Here's how the part is built. I have some questions about the finished solid (model axes, mm). A direction names the side the tool comes from. Round coordinates to 2 decimals unless told otherwise and drop trailing zeros. Order: outer loops, then holes, each group sorted by start corner. A loop starts at its lowest first (then second) coordinate and runs counter-clockwise, first axis right, second up. Notation, with made-up numbers: M 29.5,-16 L 67.5,-16 A17 ccw 67.5,10 Z; hole C -39.75,21 d6. An arc over 180 degrees is marked long. Write item = value, one per line. Start each with the question number.
Item 1: I'm going to push flat-ended pins straight in: P1, Ø6, axis at x = 5, y = 16.5, coming from the -Z side; P2, Ø5.5, axis at x = 0.5, y = 2, coming from the +Z side; P3, Ø5.5, axis at x = -1, z = -1.5, coming from the -Y side. Where does each tip first touch, or does it pass through?
Item 2: Please list where these lines run through material, in increasing order: L1, parallel to X at y = 16.25, z = 0 (3 decimals); L2, parallel to Z at x = -20.5, y = 2; L3, parallel to Y at x = 4, z = -19.
Item 3: For faces 1 (the face through (-2.76, 16.94, -8.75)), 2 (the face through (0, 2, 5.556)), 3 (the face through (-20, 5, 15)), which set-ups out of +Z, -Z, +X, -X, +Y, -Y let a thin tool reach every point of the face, with its end or its side?
Item 4: I want a section at B-B, the plane y = 1.75. List the corners of the cut face in (x, z) for me, plus the area to 3 significant figures.
Item 5: I want a section at A-A, the plane x = 0. List the corners of the cut face in (y, z) for me (3 decimals), plus the area to 3 significant figures.
Item 6: We'd pull the mould along X, two halves only. Please class faces 4 (the face through (-12.276, 5.07, 17.039)), 5 (the face through (-7.549, 8.683, 23.056)), 6 (the face through (19.66, 8.68, -14.22)): pulls with the +X half, pulls with the -X half, needs draft (parallel to the pull), parting line crosses it, or undercut.
Item 7: I want a section at D-D, the plane y = 12. List the corners of the cut face in (x, z) for me (3 decimals), plus the area to 3 significant figures.
Item 8: I want a section at C-C, the plane y = 19.5. List the corners of the cut face in (x, z) for me (3 decimals), plus the area to 3 significant figures.
```python
from build123d import *
from OCP.BRepFilletAPI import BRepFilletAPI_MakeChamfer

# Parameters (mm, degrees)
CUT_EXTRUDE3_DEPTH = 38.027017163
CHAMFER1_SIZE      = 1.5
CHAMFER1_SIZE2     = 2.598076211
CIRPATTERN1_COUNT  = 10
CUT_EXTRUDE2_DEPTH = 5


with BuildPart() as part:
    # Sketch1 → Revolve1 (revolve)
    with BuildSketch(Plane.XY, mode=Mode.PRIVATE) as revolve1_sk:
        with BuildLine():
            Line((3.175, 0), (3.175, 21))
            Line((3.175, 21), (9.175, 21))
            Line((9.175, 21), (9.175, 13))
            ThreePointArc((9.175, 13), (10.053679656, 10.878679656), (12.175, 10))
            Line((12.175, 10), (25, 10))
            Line((25, 10), (25, 0))
            Line((25, 0), (3.175, 0))
        make_face()
    revolve(revolve1_sk.sketch.rotate(Axis((0, 0, 0), (0, 1, 0)), 90), axis=Axis((0, 0, 0), (0, 1, 0)))

    # Sketch4 → Cut-Extrude3 (cut, through all)
    with BuildSketch(Plane(origin=(0, 10, 0), x_dir=(1, 0, 0), z_dir=(0, 1, 0))):
        with BuildLine():
            ThreePointArc((-3.987179454, 24.68), (0, 21), (3.987179454, 24.68))
            ThreePointArc((3.987179454, 24.68), (0, 25), (-3.987179454, 24.68))
        make_face()
    cut_extrude3 = extrude(amount=-CUT_EXTRUDE3_DEPTH, mode=Mode.SUBTRACT)

    # Chamfer1: one chamfer whose edges measure the first distance from different faces: ONE call of the kernel's chamfer builder (chamfer() names one face for all edges)
    chamfer1_edges_1 = [part.edges().sort_by_distance(p)[0] for p in [
        (0, 10, 25),
    ]]
    chamfer1_side_1 = [part.faces().sort_by_distance(p)[0] for p in [
        (0, 10, 24.295152329),
    ]]
    chamfer1_edges_2 = [part.edges().sort_by_distance(p)[0] for p in [
        (0, 0, 25),
    ]]
    chamfer1_side_2 = [part.faces().sort_by_distance(p)[0] for p in [
        (0, 0, -20.295152329),
    ]]
    chamfer1 = BRepFilletAPI_MakeChamfer(part.part.solid().wrapped)
    for e in chamfer1_edges_1:
        chamfer1.Add(CHAMFER1_SIZE, CHAMFER1_SIZE2, e.wrapped, chamfer1_side_1[0].wrapped)  # the first distance lies on this face
    for e in chamfer1_edges_2:
        chamfer1.Add(CHAMFER1_SIZE, CHAMFER1_SIZE2, e.wrapped, chamfer1_side_2[0].wrapped)  # the first distance lies on this face
    add(Compound.cast(chamfer1.Shape()), mode=Mode.REPLACE)

    # CirPattern1: Cut-Extrude3 ×10 about axis
    cirpattern1_axis = Axis((0, 0, 0), (0, 1, 0))
    for i in range(1, CIRPATTERN1_COUNT):
        add(cut_extrude3.rotate(cirpattern1_axis, i * 360 / CIRPATTERN1_COUNT), mode=Mode.SUBTRACT)

    # Sketch3 → Cut-Extrude2 (cut)
    with BuildSketch(Plane.XZ):
        Polygon((3.207902433, 5.55625), (-3.207902433, 5.55625), (-6.415804866, 0), (-3.207902433, -5.55625), (3.207902433, -5.55625), (6.415804866, 0), align=None)
    extrude(amount=-CUT_EXTRUDE2_DEPTH, mode=Mode.SUBTRACT)


solid = part.part
```
Filled in:
q1.P1 = -8.95
q1.P2 = 22.67
q1.P3 = 5
q2.L1 = -9.175 to -3.175, 3.175 to 9.175
q2.L2 = -13.7 to -10.02, -5.43 to 5.43, 10.02 to 13.7
q2.L3 = 0 to 10
q3.face_1 = +Y
q3.face_2 = -Y
q3.face_3 = +Z, -X, +Y, -Y
q4.outline = M -24.22,-3.75 A4 cw -21.8,-11.2 A24.51 ccw -17.39,-17.27 A4 cw -11.05,-21.88 A24.51 ccw -3.92,-24.2 A4 cw 3.92,-24.2 A24.51 ccw 11.05,-21.88 A4 cw 17.39,-17.27 A24.51 ccw 21.8,-11.2 A4 cw 24.22,-3.75 A24.51 ccw 24.22,3.75 A4 cw 21.8,11.2 A24.51 ccw 17.39,17.27 A4 cw 11.05,21.88 A24.51 ccw 3.92,24.2 A4 cw -3.92,24.2 A24.51 ccw -11.05,21.88 A4 cw -17.39,17.27 A24.51 ccw -21.8,11.2 A4 cw -24.22,3.75 A24.51 ccw Z; hole M -6.42,0 L -3.21,-5.56 L 3.21,-5.56 L 6.42,0 L 3.21,5.56 L -3.21,5.56 Z
q4.area = 1,580 mm^2
q5.outline = M 0,-21 L 10,-21 L 10,-12.175 A3 cw 13,-9.175 L 21,-9.175 L 21,-3.175 L 5,-3.175 L 5,-5.556 L 0,-5.556 Z; M 0,5.556 L 5,5.556 L 5,3.175 L 21,3.175 L 21,9.175 L 13,9.175 A3 cw 10,12.175 L 10,21 L 0,21 Z
q5.area = 469 mm^2
q6.face_4 = undercut
q6.face_5 = pulls with the -X half
q6.face_6 = pulls with the +X half
q7.outline = C 0,0 d18.693; hole C 0,0 d6.35
q7.area = 243 mm^2
q8.outline = C 0,0 d18.35; hole C 0,0 d6.35
q8.area = 233 mm^2
